Model file for the job. Use its own axes, mm. Face numbers are marked on the shaded views. A direction names the side the tool comes from. Give positions to 0.01 mm unless a question says otherwise; leave off trailing zeros. Order: outer loops, then holes, each group sorted by start corner. A loop starts at its lowest first (then second) coordinate and runs counter-clockwise, first axis right, second up. Notation, with made-up numbers: M 88.5,81 L 133.5,81 A12 ccw 133.5,91 Z; hole C 34.5,69.5 d8. An arc over 180 degrees is marked long. Return JSON: item names as keys, results as strings. Group by question number.
1. Wall check: probe 1 along X at (y, z) = (-1, 1.75); probe 2 along X at (y, z) = (-0.75, 1.9); probe 3 along Z at (x, y) = (-8.5, 0.75). Give the ranges that are in metal, low to high. Write a range as [from, to].
2. 3-axis set-ups, long thin cutter, end or side, ignore diameter. For the marked faces 1 and 2: which of +Z, -Z, +X, -X, +Y, -Y reach the whole face in a straight line?
3. Slice it at B-B on z = 1.9. List the corners of the cut face in (x, y), then the cut area to 3 significant figures.
4. Slice it at C-C on x = -10.5. List the corners of the cut face in (y, z).
5. Slice it at A-A on y = -1. List the corners of the cut face in (x, z), then the cut area to 3 significant figures.
6. Slice it at D-D on x = -5.5. List the corners of the cut face in (y, z).
7. Pin check, flat tips, straight feed: pin 1 (6 mm diameter, centred on x = -4.5, y = -1.5, fed in from +Z); pin 2 (4 mm diameter, centred on x = -5.461, y = 0, fed in from -Z); pin 3 (4.5 mm diameter, centred on x = 2.48, y = 0, fed in from +Z); pin 4 (1.5 mm diameter, centred on x = 4.5, z = -0.5, fed in from -Y). Stop position of each tip, or through.
8. Two-plate mould, pull along X, no slides. Class the marked faces 3, 4, 5 and 6: released by +X, released by -X, zero draft, split by the parting line, or undercut.
from build123d import *

# Parameters (mm, degrees)
SKETCH2_W                  = 31.75
SKETCH2_H                  = 10.16
SKETCH2_R                  = 1.4732
BOSS_EXTRUDE1_DEPTH        = 2.54
F_6_0_204_DIAMETER_HOLE1_D = 5.1816
SKETCH5_W                  = 7.62
SKETCH5_H                  = 4.572
BOSS_EXTRUDE2_DEPTH        = 0.254
SKETCH6_R                  = 0.381
CUT_EXTRUDE1_DEPTH         = 3.794
SKETCH7_R                  = 3.683
BOSS_EXTRUDE3_DEPTH        = 2.032


with BuildPart() as part:
    # Sketch2 → Boss-Extrude1 (new body)
    with BuildSketch(Plane.XY):
        with Locations((-0.381, 0)):
            Rectangle(SKETCH2_W, SKETCH2_H)
        with Locations((-5.461, 0)):
            Circle(SKETCH2_R, mode=Mode.SUBTRACT)
        with Locations((10.414, 0)):
            Circle(SKETCH2_R, mode=Mode.SUBTRACT)
    extrude(amount=BOSS_EXTRUDE1_DEPTH)

    # #6 (0.204) Diameter Hole1 (through all)
    with Locations(Plane(origin=(2.4765, 0, 2.54), x_dir=(1, 0, 0), z_dir=(0, 0, 1))):
        with Locations((0, 0)):
            Hole(F_6_0_204_DIAMETER_HOLE1_D / 2)

    # Sketch5 → Boss-Extrude2 (add)
    with BuildSketch(Plane.XY.offset(2.54)):
        with Locations((-12.192, 2.413)):
            Rectangle(SKETCH5_W, SKETCH5_H)
        with Locations((-12.192, -2.413)):
            Rectangle(SKETCH5_W, SKETCH5_H)
    extrude(amount=BOSS_EXTRUDE2_DEPTH)

    # Sketch6 → Cut-Extrude1 (cut, through all)
    with BuildSketch(Plane.XY.offset(2.794)):
        with Locations((-12.192, 2.413)):
            Circle(SKETCH6_R)
        with Locations((-12.192, -2.413)):
            Circle(SKETCH6_R)
    extrude(amount=-CUT_EXTRUDE1_DEPTH, mode=Mode.SUBTRACT)

    # Sketch7 → Boss-Extrude3 (add)
    with BuildSketch(Plane(origin=(0, 0, 0), x_dir=(-1, 0, 0), z_dir=(0, 0, -1))):
        with Locations((-2.4765, 0)):
            Circle(SKETCH7_R)
    extrude(amount=BOSS_EXTRUDE3_DEPTH)


solid = part.part
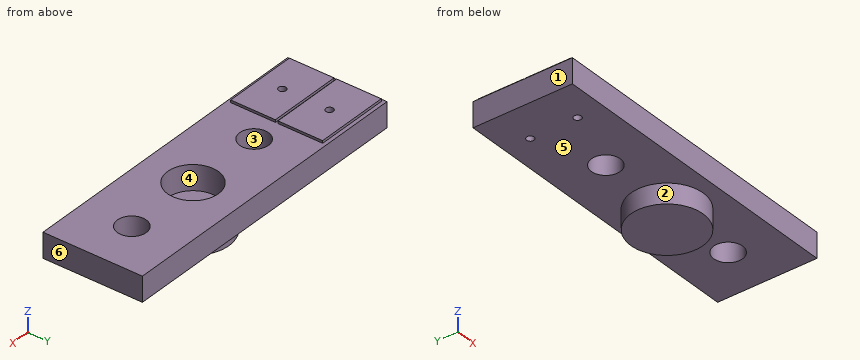
Result:
{
 "1": {"probe 1": "x = [-16.26, -6.54], [-4.38, 0.09], [4.87, 9.33], [11.5, 15.49]", "probe 2": "x = [-16.26, -6.73], [-4.19, 0], [4.96, 9.15], [11.68, 15.49]", "probe 3": "z = [0, 2.79]"},
 "2": {"face 1": "+Z, -Z, -X, +Y, -Y", "face 2": "-Z"},
 "3": {"outline": "M -16.26,-5.08 L 15.49,-5.08 L 15.49,5.08 L -16.26,5.08 Z; hole C -12.19,-2.41 d0.76; hole C -12.19,2.41 d0.76; hole C -5.46,0 d2.95; hole C 2.48,0 d5.18; hole C 10.41,0 d2.95", "area": "287 mm2"},
 "4": {"outline": "M -5.08,0 L 5.08,0 L 5.08,2.54 L 4.7,2.54 L 4.7,2.79 L 0.13,2.79 L 0.13,2.54 L -0.13,2.54 L -0.13,2.79 L -4.7,2.79 L -4.7,2.54 L -5.08,2.54 Z"},
 "5": {"outline": "M -16.26,0 L -6.54,0 L -6.54,2.54 L -8.38,2.54 L -8.38,2.79 L -16,2.79 L -16,2.54 L -16.26,2.54 Z; M -4.38,0 L -1.07,0 L -1.07,-2.03 L 6.02,-2.03 L 6.02,0 L 9.33,0 L 9.33,2.54 L 4.87,2.54 L 4.87,0 L 0.09,0 L 0.09,2.54 L -4.38,2.54 Z; M 11.5,0 L 15.49,0 L 15.49,2.54 L 11.5,2.54 Z", "area": "73.9 mm2"},
 "6": {"outline": "M -5.08,0 L -1.47,0 L -1.47,2.54 L -5.08,2.54 Z; M 1.47,0 L 5.08,0 L 5.08,2.54 L 1.47,2.54 Z"},
 "7": {"pin 1": "stops at z = 2.54", "pin 2": "stops at z = 0", "pin 3": "stops at z = 0", "pin 4": "stops at y = -5.08"},
 "8": {"face 3": "undercut", "face 4": "undercut", "face 5": "zero draft", "face 6": "released by +X"}
}
